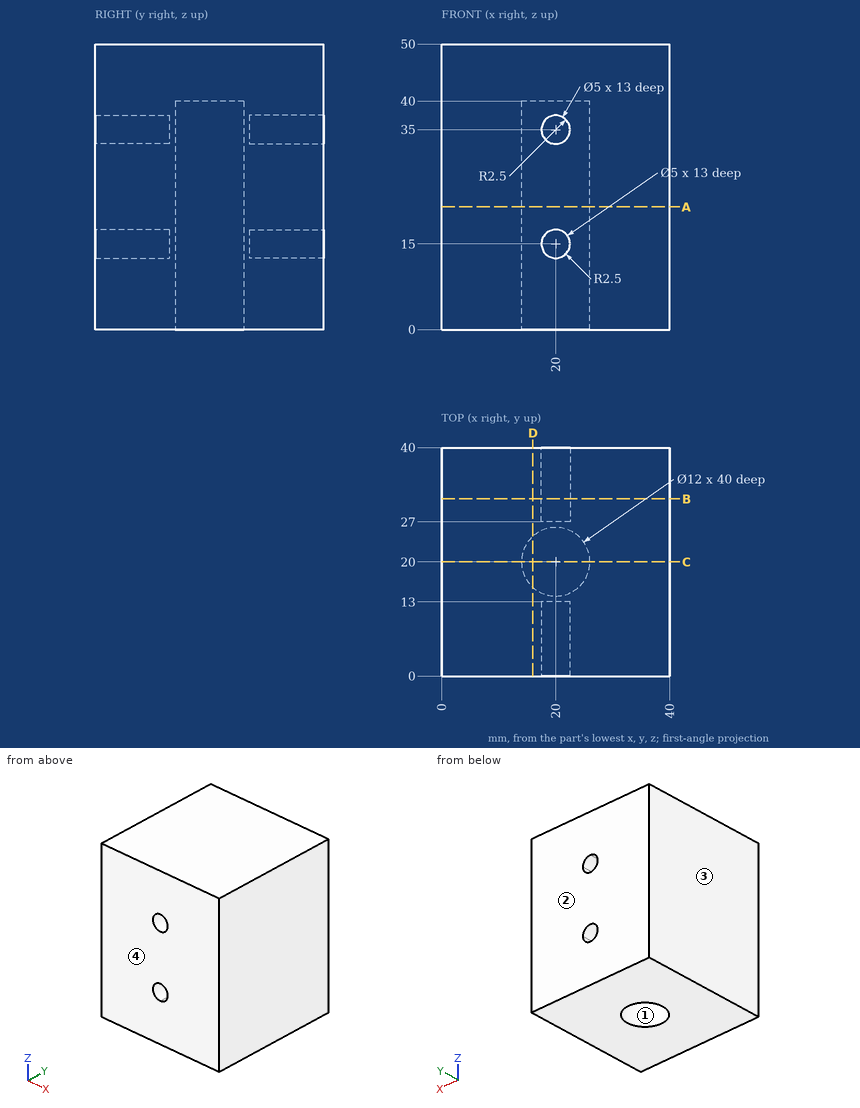
Geometry check sheet. Reference: drawing and pictorial views, mm from the part's lowest x, y, z. Round coordinates to 2 decimals unless told otherwise and drop trailing zeros. Loops run counter-clockwise (first coordinate to the right, second up) from the corner with the lowest first, then second, coordinate; pieces in that order, holes last. Notation, with made-up numbers: (-26.5, 23) - (6.5, 23) arc R27 cw to (6.5, 50) - close; hole circle Ø3 at (76.25, 50.5). An arc over 180 degrees is marked (long way). Answer in a Markdown table with one row per item. Add a question column.
Q1. Section check B-B on y = 31. Enter the section's corners in (x, z).
Q2. Material ranges on line 1 (Z direction, x = 20, y = 30.5); line 2 (X direction, y = 9.75, z = 35); line 3 (Y direction, x = 20, z = 7), recorded low to high.
Q3. Gauge pin test, flat ends, axial feed: pin 1 (3.5 mm diameter, centred on x = 21.5, y = 19.5, fed in from -Z); pin 2 (4 mm diameter, centred on x = 20, z = 15, fed in from -Y); pin 3 (1 mm diameter, centred on x = 12.5, z = 5.5, fed in from -Y); pin 4 (1.5 mm diameter, centred on x = 19.5, z = 34.5, fed in from +Y). Record the tip position at first contact, or that the pin passes through.
Q4. Section check A-A on z = 21.5. Enter the section's corners in (x, y), plus the area to 3 significant figures.
Q5. Section check D-D on x = 16. Enter the section's corners in (y, z).
Q6. Section check C-C on y = 20. Enter the section's corners in (x, z), plus the area to 3 significant figures.
Q7. Release check for a two-part mould opening along Y. For the marked faces 1, 2, 3 and 4 record: pulls with the +Y half, pulls with the -Y half, needs draft (parallel to the pull), parting line crosses it, or undercut.
Found:
| question | item | result |
|---|---|---|
| 1 | outline | (0, 0) - (40, 0) - (40, 50) - (0, 50) - close; hole circle Ø5 at (20, 15); hole circle Ø5 at (20, 35) |
| 2 | line 1 | z = 0 to 12.5, 17.5 to 32.5, 37.5 to 50 |
| 2 | line 2 | x = 0 to 17.5, 22.5 to 40 |
| 2 | line 3 | y = 0 to 14, 26 to 40 |
| 3 | pin 1 | stops at z = 40 |
| 3 | pin 2 | stops at y = 13 |
| 3 | pin 3 | stops at y = 0 |
| 3 | pin 4 | stops at y = 27 |
| 4 | outline | (0, 0) - (40, 0) - (40, 40) - (0, 40) - close; hole circle Ø12 at (20, 20) |
| 4 | area | 1,490 mm² |
| 5 | outline | (0, 0) - (15.53, 0) - (15.53, 40) - (24.47, 40) - (24.47, 0) - (40, 0) - (40, 50) - (0, 50) - close |
| 6 | outline | (0, 0) - (14, 0) - (14, 40) - (26, 40) - (26, 0) - (40, 0) - (40, 50) - (0, 50) - close |
| 6 | area | 1,520 mm² |
| 7 | face 1 | undercut |
| 7 | face 2 | pulls with the +Y half |
| 7 | face 3 | needs draft |
| 7 | face 4 | pulls with the -Y half |
